```python
from build123d import *

# Parameters (mm, degrees)
SKETCH1_W           = 30
SKETCH1_H           = 37.5
BOSS_EXTRUDE1_DEPTH = 3
SKETCH2_W           = 3
SKETCH2_H           = 15
BOSS_EXTRUDE2_DEPTH = 3
SKETCH3_R           = 1.85
CUT_EXTRUDE1_DEPTH  = 27.164145314
SKETCH4_W           = 15.1
SKETCH4_H           = 3.1
CUT_EXTRUDE2_DEPTH  = 27.164145314


with BuildPart() as part:
    # Sketch1 → Boss-Extrude1 (new body)
    with BuildSketch(Plane(origin=(0, 0, 0), x_dir=(1, 0, 0), z_dir=(0, 1, 0))):
        Rectangle(SKETCH1_W, SKETCH1_H)
    extrude(amount=BOSS_EXTRUDE1_DEPTH)

    # Sketch2 → Boss-Extrude2 (add)
    with BuildSketch(Plane(origin=(0, 3, 0), x_dir=(1, 0, 0), z_dir=(0, 1, 0))):
        with Locations((-16.5, 0)):
            Rectangle(SKETCH2_W, SKETCH2_H)
        with Locations((16.5, 0)):
            Rectangle(SKETCH2_W, SKETCH2_H)
    extrude(amount=-BOSS_EXTRUDE2_DEPTH)

    # Sketch3 → Cut-Extrude1 (cut, through all)
    with BuildSketch(Plane(origin=(0, 3, 0), x_dir=(1, 0, 0), z_dir=(0, 1, 0))):
        with Locations((-16.5, 0)):
            Circle(SKETCH3_R)
        with Locations((16.5, 0)):
            Circle(SKETCH3_R)
    extrude(amount=-CUT_EXTRUDE1_DEPTH, mode=Mode.SUBTRACT)

    # Sketch4 → Cut-Extrude2 (cut, through all)
    with BuildSketch(Plane(origin=(0, 3, 0), x_dir=(1, 0, 0), z_dir=(0, 1, 0))):
        with Locations((0, -13.2)):
            Rectangle(SKETCH4_W, SKETCH4_H)
    extrude(amount=-CUT_EXTRUDE2_DEPTH, mode=Mode.SUBTRACT)


solid = part.part
```
Could you check a few things on this model? Use its own coordinates, in mm. A direction names the side the tool comes from. Give positions to 0.01 mm unless a question says otherwise; leave off trailing zeros. Order: outer loops, then holes, each group sorted by start corner. A loop starts at its lowest first (then second) coordinate and runs counter-clockwise, first axis right, second up.
Q1. Suppose I cut it at D-D, the plane z = -9.5. Write out the boundary of the cut face in (x, y).
Q2. Suppose I cut it at B-B, the plane z = 13.5. Write out the boundary of the cut face in (x, y), and give its area (3 significant figures).
Q3. Suppose I cut it at C-C, the plane y = 1.65. Write out the boundary of the cut face in (x, z).
Q4. I'm going to push flat-ended pins straight in: P1, Ø1.5, axis at x = -16.5, y = 2, coming from the -Z side; P2, Ø2, axis at x = -16.5, z = 0, coming from the -Y side; P3, Ø1.5, axis at y = 1.5, z = -15, coming from the -X side; P4, Ø3, axis at x = -10.5, z = 12.5, coming from the -Y side. Where does each tip first touch, or does it pass through?
Q5. If I drill on line 1 along X through (y, z) = (1.55, 12.5); line 2 along Z through (x, y) = (6, 0.2); line 3 along Z through (x, y) = (-16.5, 1.7), over which ranges is the centre line in solid material (lowest first)?
Q6. For faces 1 (the flat face through (16, 2, -7.5)), 2 (the flat face through (-17, 2, -7.5)), 3 (the flat face through (15, 1, 13)), which set-ups out of +Z, -Z, +X, -X, +Y, -Y let a thin tool reach every point of the face, with its end or its side?
Q7. Suppose I cut it at A-A, the plane x = 1. Write out the boundary of the cut face in (y, z).
Solution:
1. outline: (-15, 0) - (15, 0) - (15, 3) - (-15, 3) - close
2. outline: (-15, 0) - (-7.55, 0) - (-7.55, 3) - (-15, 3) - close; (7.55, 0) - (15, 0) - (15, 3) - (7.55, 3) - close
2. area: 44.7 mm2
3. outline: (-18, -7.5) - (-15, -7.5) - (-15, -18.75) - (15, -18.75) - (15, -7.5) - (18, -7.5) - (18, -1.08) arc R1.85 cw (long way) to (18, 1.08) - (18, 7.5) - (15, 7.5) - (15, 18.75) - (-15, 18.75) - (-15, 7.5) - (-18, 7.5) - (-18, 1.08) arc R1.85 cw (long way) to (-18, -1.08) - close; hole (-7.55, 11.65) - (7.55, 11.65) - (7.55, 14.75) - (-7.55, 14.75) - close
4. P1: stops at z = -7.5
4. P2: passes through
4. P3: stops at x = -15
4. P4: stops at y = 0
5. line 1: x = -15 to -7.55, 7.55 to 15
5. line 2: z = -18.75 to 11.65, 14.75 to 18.75
5. line 3: z = -7.5 to -1.85, 1.85 to 7.5
6. face 1: -Z, +X, +Y, -Y
6. face 2: -Z, -X, +Y, -Y
6. face 3: +Z, +X, +Y, -Y
7. outline: (0, -18.75) - (3, -18.75) - (3, 11.65) - (0, 11.65) - close; (0, 14.75) - (3, 14.75) - (3, 18.75) - (0, 18.75) - close
